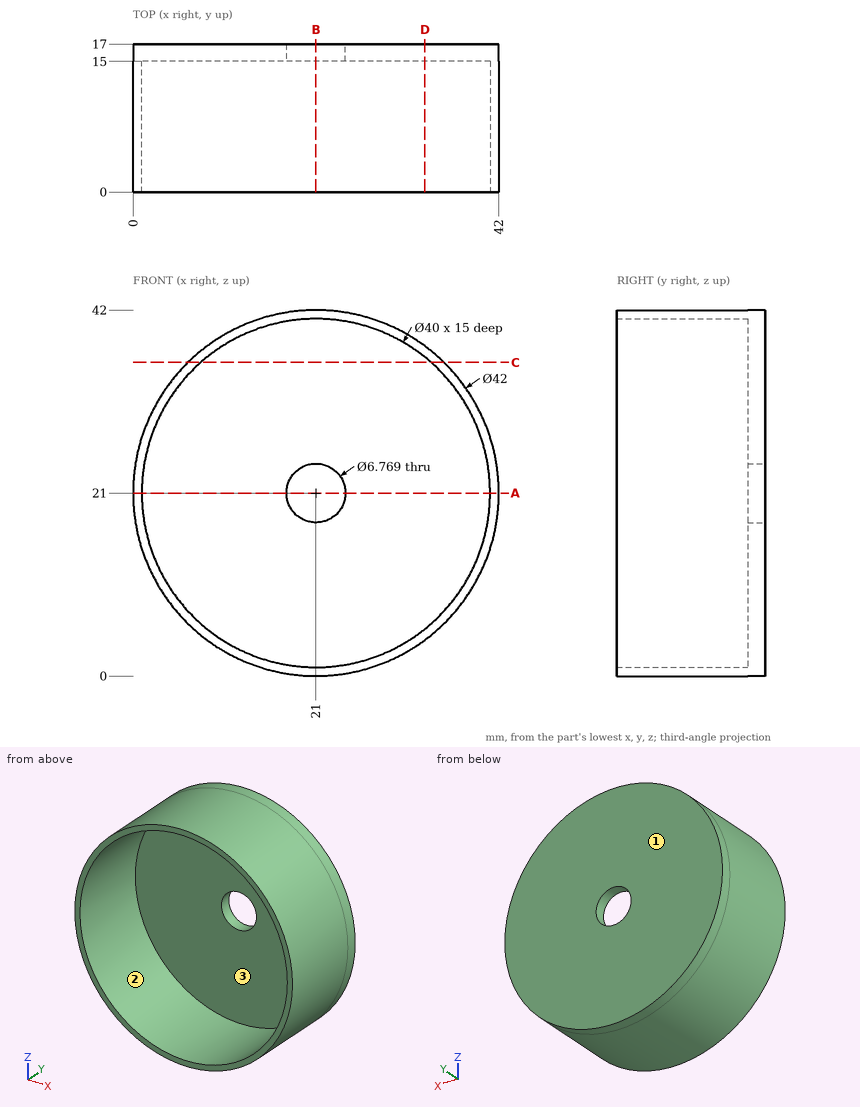
Could you check a few things on this drawing? It's one solid part, dimensions in mm from its lowest x, y, z. Coordinates: 2 decimals unless noted, no trailing zeros. Order: outer loops, then holes, each group sorted by start corner. A loop starts at its lowest first (then second) coordinate and runs counter-clockwise, first axis right, second up. Notation, with made-up numbers: (28, -7.75) - (60, -7.75) arc R26 ccw to (60, 7.25) - close; hole circle Ø3 at (31.25, 62.25). An arc over 180 degrees is marked (long way). Answer as a JSON object with one key per item and string values. Group by question number.
Q1. Imagine slicing it at C-C (z = 36). Please give me the cut outline in (x, y), and give its area (3 significant figures).
Q2. We'd pull the mould along X, two halves only. Please class the marked faces 1, 2 and 3: +X half, -X half, draft (parallel to the pull), parting line (faces both ways), or undercut.
Q3. Imagine slicing it at D-D (x = 33.5). Please give me the cut outline in (y, z), and give its area (3 significant figures).
Q4. Will these pins go through, and if not, where does the flat tip stop? P1, Ø8, axis at y = 5, z = 36.5, coming from the -X side; P2, Ø4, axis at x = 26, y = 11.5, coming from the -Z side; P3, Ø8, axis at x = 11.5, y = 2.5, coming from the +Z side; P4, Ø4, axis at x = 21, z = 21, coming from the +Y side.
Q5. Imagine slicing it at B-B (x = 21). Please give me the cut outline in (y, z).
Q6. Imagine slicing it at A-A (z = 21). Please give me the cut outline in (x, y), and give its area (3 significant figures).
Q7. I need wall thicknesses on line 1 (Z direction, x = 21, y = 15.65); line 2 (Z direction, x = 21, y = 11); line 3 (Y direction, x = 13.5, z = 5). Which ranges of each line are inside material? Lowest first, please. Write a range as from..to.
Determined:
{
 "1": {"outline": "(6.3, 0) - (7.77, 0) - (7.77, 15) - (34.23, 15) - (34.23, 0) - (35.7, 0) - (35.7, 17) - (6.3, 17) - close", "area": "103 mm2"},
 "2": {"face 1": "draft", "face 2": "undercut", "face 3": "undercut"},
 "3": {"outline": "(0, 4.13) - (17, 4.13) - (17, 37.87) - (0, 37.87) - (0, 36.61) - (15, 36.61) - (15, 5.39) - (0, 5.39) - close", "area": "105 mm2"},
 "4": {"P1": "stops at x = 3.43", "P2": "stops at z = 0.22", "P3": "stops at z = 41.27", "P4": "passes through"},
 "5": {"outline": "(0, 0) - (17, 0) - (17, 17.62) - (15, 17.62) - (15, 1) - (0, 1) - close; (0, 41) - (15, 41) - (15, 24.38) - (17, 24.38) - (17, 42) - (0, 42) - close"},
 "6": {"outline": "(0, 0) - (1, 0) - (1, 15) - (17.62, 15) - (17.62, 17) - (0, 17) - close; (24.38, 15) - (41, 15) - (41, 0) - (42, 0) - (42, 17) - (24.38, 17) - close", "area": "100 mm2"},
 "7": {"line 1": "z = 0..17.62, 24.38..42", "line 2": "z = 0..1, 41..42", "line 3": "y = 15..17"}
}
